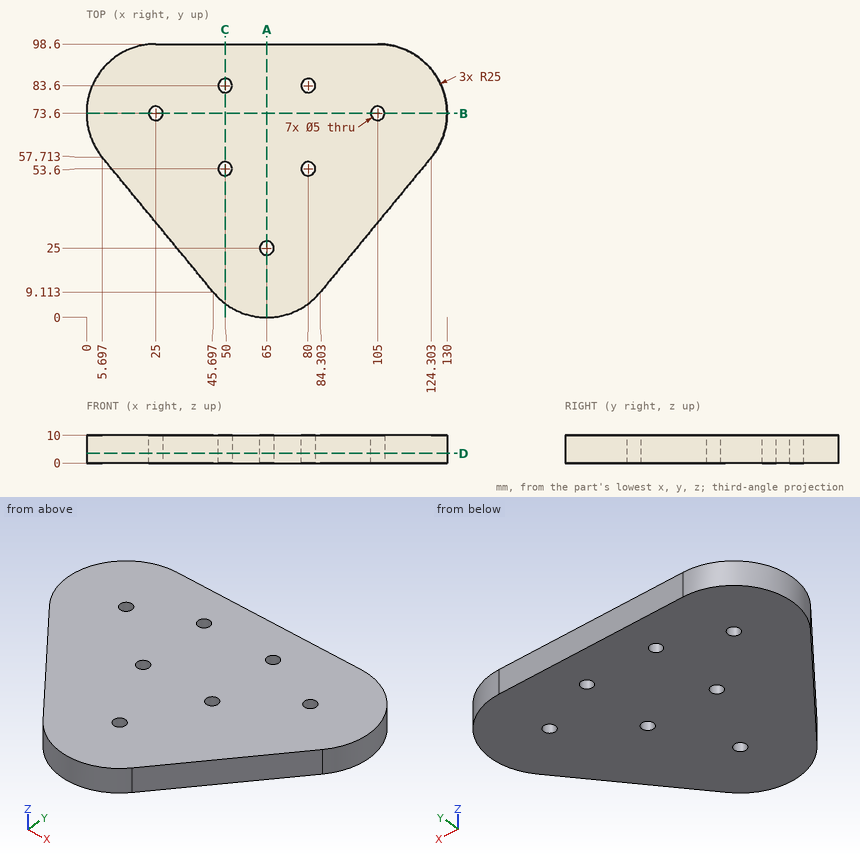
The drawing under review shows one solid part. Ordinate dimensions are in mm from its lowest x, y, z. Round coordinates to 2 decimals unless told otherwise and drop trailing zeros. Write each loop counter-clockwise with the first axis right and the second up, starting at its lowest first coordinate (ties: lowest second). Pieces come first, ordered by that corner, then holes. Notation, with made-up numbers: (-9.75, -14.5) - (17.25, -14.5) arc R25 ccw to (17.25, 24.5) - close; hole circle Ø7 at (29, 46.5). An arc over 180 degrees is marked (long way). Put each result on its own line as item: value.
Q1. We need section B-B (y = 73.6). Give the boundary of the cut face in (x, z).
Solved:
outline: (0, 0) - (22.5, 0) - (22.5, 10) - (0, 10) - close; (27.5, 0) - (102.5, 0) - (102.5, 10) - (27.5, 10) - close; (107.5, 0) - (130, 0) - (130, 10) - (107.5, 10) - close
Q2. Insertion check: pin 1 Ø3 at (x, z) = (49, 6) entering from -Y (1 decimal); pin 2 Ø5 at (x, y) = (82, 47) entering from -Z; pin 3 Ø6 at (x, z) = (103.5, 6) entering from -Y; pin 4 Ø1 at (y, z) = (35.5, 2.5) entering from -X. Each pin has a flat end and moves straight along its axis. Give the tip position at first contact, or say it passes through.
Solved:
pin 1: stops at y = 4.6
pin 2: stops at z = 0
pin 3: stops at y = 28.79
pin 4: stops at x = 23.57
Q3. Wall thickness on probe 1 along Y at (x, z) = (50, 4.25); probe 2 along Y at (x, z) = (48.5, 8.5); probe 3 along X at (y, z) = (52.5, 1.5) (1 decimal): over which ranges is each line inside the solid? List them lowest first.
Solved:
probe 1: y = 5 to 51.1, 56.1 to 81.1, 86.1 to 98.6
probe 2: y = 6.22 to 51.6, 55.6 to 81.6, 85.6 to 98.6
probe 3: x = 10 to 47.8, 52.2 to 77.8, 82.2 to 120
Q4. We need section C-C (x = 50). Give the boundary of the cut face in (y, z), and give its area (3 significant figures).
Solved:
outline: (5, 0) - (51.1, 0) - (51.1, 10) - (5, 10) - close; (56.1, 0) - (81.1, 0) - (81.1, 10) - (56.1, 10) - close; (86.1, 0) - (98.6, 0) - (98.6, 10) - (86.1, 10) - close
area: 836 mm2
Q5. We need section A-A (x = 65). Give the boundary of the cut face in (y, z), and give its area (3 significant figures).
Solved:
outline: (0, 0) - (22.5, 0) - (22.5, 10) - (0, 10) - close; (27.5, 0) - (98.6, 0) - (98.6, 10) - (27.5, 10) - close
area: 936 mm2
Q6. We need section D-D (z = 3.5). Give the boundary of the cut face in (x, y).
Solved:
outline: (5.7, 57.71) - (45.7, 9.11) arc R25 ccw to (84.3, 9.11) - (124.3, 57.71) arc R25 ccw to (105, 98.6) - (25, 98.6) arc R25 ccw to start; hole circle Ø5 at (25, 73.6); hole circle Ø5 at (50, 53.6); hole circle Ø5 at (50, 83.6); hole circle Ø5 at (65, 25); hole circle Ø5 at (80, 53.6); hole circle Ø5 at (80, 83.6); hole circle Ø5 at (105, 73.6)
